from build123d import *

# Parameters (mm, degrees)
SKETCH_W          = 35
SKETCH_H          = 20
PAD_DEPTH         = 20
SKETCH001_W       = 30
SKETCH001_H       = 15
POCKET_DEPTH      = 0.001
POCKET_DEPTH_BACK = 20.001
SKETCH002_R       = 3.75
POCKET001_DEPTH   = 3.5
SKETCH003_R       = 1.875
POCKET002_DEPTH   = 2.5
CHAMFER_SIZE      = 2.485
FILLET_R          = 1


with BuildPart() as part:
    # Sketch → Pad (new body)
    with BuildSketch(Plane.XZ):
        Rectangle(SKETCH_W, SKETCH_H)
    extrude(amount=PAD_DEPTH)

    # Sketch001 → Pocket (cut, two sides)
    with BuildSketch(Plane.XZ) as pocket_sk:
        Rectangle(SKETCH001_W, SKETCH001_H)
    extrude(amount=-POCKET_DEPTH, mode=Mode.SUBTRACT)
    extrude(pocket_sk.sketch, amount=POCKET_DEPTH_BACK, mode=Mode.SUBTRACT)

    # Sketch002 (on DatumPlane) → Pocket001 (cut)
    with BuildSketch(Plane(origin=(0, 0, 10), x_dir=(-1, 0, 0), z_dir=(0, 0, 1))):
        with Locations((-8.125, 10)):
            Circle(SKETCH002_R)
        with Locations((8.125, 10)):
            Circle(SKETCH002_R)
    extrude(amount=-POCKET001_DEPTH, mode=Mode.SUBTRACT)

    # Sketch003 (on DatumPlane) → Pocket002 (cut)
    with BuildSketch(Plane(origin=(0, 0, -7.5), x_dir=(-1, 0, 0), z_dir=(0, 0, 1))):
        with Locations((-8.125, 10)):
            Circle(SKETCH003_R)
        with Locations((8.125, 10)):
            Circle(SKETCH003_R)
    extrude(amount=-POCKET002_DEPTH, mode=Mode.SUBTRACT)

    # Chamfer
    chamfer_edges = [part.edges().sort_by_distance(p)[0] for p in [
        (-6.25, -10, -7.5),
        (10, -10, -7.5),
    ]]
    chamfer(chamfer_edges, length=CHAMFER_SIZE)

    # Fillet
    fillet_edges = [part.edges().sort_by_distance(p)[0] for p in [
        (-17.5, -20, 0),
        (0, -20, 10),
        (0, -20, -10),
        (17.5, -20, 0),
        (-15, -20, 0),
        (0, -20, 7.5),
        (15, -20, 0),
        (0, -20, -7.5),
        (-4.375, -10, 10),
        (11.875, -10, 10),
        (17.5, -10, 10),
        (17.5, -10, -10),
        (-17.5, 0, 0),
        (0, 0, 10),
        (0, 0, -10),
        (17.5, 0, 0),
        (-15, 0, 0),
        (0, 0, 7.5),
        (15, 0, 0),
        (0, 0, -7.5),
    ]]
    fillet(fillet_edges, radius=FILLET_R)


solid = part.part
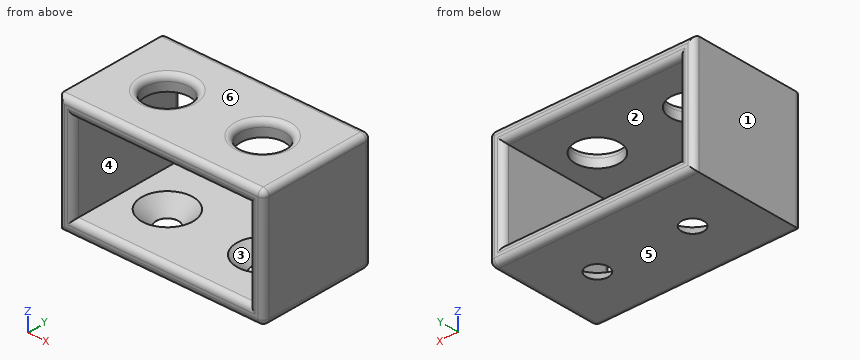
Work out the finished part from the listing and answer in its coordinate system (mm). Face numbers are marked on the shaded views. A direction names the side the tool comes from. Give positions to 0.01 mm unless a question says otherwise; leave off trailing zeros. Loops run counter-clockwise (first coordinate to the right, second up) from the corner with the lowest first, then second, coordinate; pieces in that order, holes last. Notation, with made-up numbers: (-33, 13) - (19, 13) arc R29 ccw to (19, 42) - close; hole circle Ø4 at (64.25, 16). An arc over 180 degrees is marked (long way). Answer in a Markdown table with one row per item.
(1) Consider L1, parallel to X at y = -10, z = 8.35 (3 decimals); L2, parallel to X at y = -14.5, z = 1.5; L3, parallel to Z at x = 2, y = -19. Determine where each line is inside the solid, lowest interval first. Write a range as [from, to].
Results list:
| item | result |
|---|---|
| L1 | x = [-17.5, -11.875], [-4.375, 4.375], [11.875, 17.5] |
| L2 | x = [-17.5, -15], [15, 17.5] |
| L3 | z = [-10, -7.5], [7.5, 10] |
(2) A tool of negligible diameter and unlimited length cuts with its end or side. For the marked faces 1, 2 and 3, from which of +Z, -Z, +X, -X, +Y, -Y can it reach the whole face along a straight path? Write none if from no direction.
Results list:
| item | result |
|---|---|
| face 1 | +Z, -Z, -X, +Y, -Y |
| face 2 | +Y, -Y |
| face 3 | none |
(3) Flat-ended cylindrical pins translate along their axes: pin 1 Ø1 at (x, z) = (3.5, -7.5) entering from +Y; pin 2 Ø4.5 at (x, y) = (8.125, -10) entering from +Z; pin 3 Ø2 at (x, z) = (12, 7) entering from -Y. Find the tip coordinate at first contact, or state that the pin passes through.
Results list:
| item | result |
|---|---|
| pin 1 | stops at y = -0.13 |
| pin 2 | stops at z = -9.61 |
| pin 3 | stops at y = -19.87 |
(4) Section B-B (x = 1) is taken. Give the vertices of the cut face in (y, z).
Results list:
| item | result |
|---|---|
| outline | (-20, -9) arc R1 ccw to (-19, -10) - (-1, -10) arc R1 ccw to (0, -9) - (0, -8.5) arc R1 ccw to (-1, -7.5) - (-19, -7.5) arc R1 ccw to (-20, -8.5) - close; (-20, 8.5) arc R1 ccw to (-19, 7.5) - (-1, 7.5) arc R1 ccw to (0, 8.5) - (0, 9) arc R1 ccw to (-1, 10) - (-19, 10) arc R1 ccw to (-20, 9) - close |
(5) For a pull along Z with two mould halves and no side action, classify the marked faces 4, 5 and 6 as pulls with the +Z half, pulls with the -Z half, needs draft (parallel to the pull), parting line crosses it, or undercut.
Results list:
| item | result |
|---|---|
| face 4 | undercut |
| face 5 | pulls with the -Z half |
| face 6 | pulls with the +Z half |
(6) Section C-C (z = 4) is taken. Give the vertices of the cut face in (x, y).
Results list:
| item | result |
|---|---|
| outline | (-17.5, -19) arc R1 ccw to (-16.5, -20) - (-16, -20) arc R1 ccw to (-15, -19) - (-15, -1) arc R1 ccw to (-16, 0) - (-16.5, 0) arc R1 ccw to (-17.5, -1) - close; (15, -19) arc R1 ccw to (16, -20) - (16.5, -20) arc R1 ccw to (17.5, -19) - (17.5, -1) arc R1 ccw to (16.5, 0) - (16, 0) arc R1 ccw to (15, -1) - close |
(7) Section D-D (z = 8) is taken. Give the vertices of the cut face in (x, y) (3 decimals).
Results list:
| item | result |
|---|---|
| outline | (-17.5, -19) arc R1 ccw to (-16.5, -20) - (-16, -20) arc R1 ccw to (-15.5, -19.866) - (15.5, -19.866) arc R1 ccw to (16, -20) - (16.5, -20) arc R1 ccw to (17.5, -19) - (17.5, -1) arc R1 ccw to (16.5, 0) - (16, 0) arc R1 ccw to (15.5, -0.134) - (-15.5, -0.134) arc R1 ccw to (-16, 0) - (-16.5, 0) arc R1 ccw to (-17.5, -1) - close; hole circle Ø7.5 at (-8.125, -10); hole circle Ø7.5 at (8.125, -10) |
(8) Section A-A (y = -10) is taken. State how many separate pieces and enclosed holes the cut face has, and give its area (3 significant figures).
Results list:
| item | result |
|---|---|
| separate pieces | 4 |
| enclosed holes | 0 |
| area | 180 mm² |
